The listing builds one solid part. Answer for the finished solid, in the listing's coordinates (mm). A direction names the side the tool comes from. Coordinates: 2 decimals unless noted, no trailing zeros. Write each loop counter-clockwise with the first axis right and the second up, starting at its lowest first coordinate (ties: lowest second). Pieces come first, ordered by that corner, then holes. Notation, with made-up numbers: M 42.25,-9 L 85.25,-9 A28 cw 85.25,10 Z; hole C -17,-17 d4. An arc over 180 degrees is marked long. Answer as CSV lines item,"result". Start each with the question number.
```python
from build123d import *

# Parameters (mm, degrees)
ESQUISSE1_R             = 5
BASE_EXTRUSION_DEPTH    = 9.5
ESQUISSE2_R             = 3.5
BOSS_EXTRU_1_DEPTH      = 0.5
ESQUISSE3_R             = 2.5
BOSS_EXTRU_2_DEPTH      = 14
ESQUISSE4_R             = 2
BOSS_EXTRU_3_DEPTH      = 12
CHANFREIN1_SIZE         = 0.5
CONG_1_R                = 0.5
ENL_V_MAT_EXTRU_1_DEPTH = 16
ESQUISSE9_R             = 1
ENL_V_MAT_EXTRU_2_DEPTH = 10


with BuildPart() as part:
    # Esquisse1 → Base-Extrusion (new body)
    with BuildSketch(Plane.XY):
        Circle(ESQUISSE1_R)
    extrude(amount=BASE_EXTRUSION_DEPTH)

    # Esquisse2 → Boss.-Extru.1 (add)
    with BuildSketch(Plane.XY.offset(9.5)):
        Circle(ESQUISSE2_R)
    extrude(amount=BOSS_EXTRU_1_DEPTH)

    # Esquisse3 → Boss.-Extru.2 (add)
    with BuildSketch(Plane.XY.offset(10)):
        Circle(ESQUISSE3_R)
    extrude(amount=BOSS_EXTRU_2_DEPTH)

    # Esquisse4 → Boss.-Extru.3 (add)
    with BuildSketch(Plane.XY.offset(24)):
        Circle(ESQUISSE4_R)
    extrude(amount=BOSS_EXTRU_3_DEPTH)

    # Chanfrein1
    chanfrein1_edges = [part.edges().sort_by_distance(p)[0] for p in [
        (-2, 0, 36),
    ]]
    chamfer(chanfrein1_edges, length=CHANFREIN1_SIZE)

    # Congé1
    cong_1_edges = [part.edges().sort_by_distance(p)[0] for p in [
        (-5, 0, 9.5),
    ]]
    fillet(cong_1_edges, radius=CONG_1_R)

    # Esquisse7 → Enlèv. mat.-Extru.1 (cut, symmetric)
    with BuildSketch(Plane(origin=(0, 0, 0), x_dir=(0, 0, -1), z_dir=(1, 0, 0))):
        with BuildLine():
            Line((1, 1.25), (-7, 1.25))
            ThreePointArc((-7, 1.25), (-8.25, 0), (-7, -1.25))
            Line((-7, -1.25), (1, -1.25))
            Line((1, -1.25), (1, 1.25))
        make_face()
    extrude(amount=ENL_V_MAT_EXTRU_1_DEPTH, both=True, mode=Mode.SUBTRACT)

    # Esquisse8 → Enlèvement de matière-Révolution1 (revolve, cut)
    with BuildSketch(Plane(origin=(0, 0, 0), x_dir=(0, 0, -1), z_dir=(1, 0, 0))):
        Polygon((0, 4.5), (-4, 3), (-8, 3), (-9.5, 0), (0, 0), align=None)
    revolve(axis=Axis((0, 0, 0), (0, 0, 1)), mode=Mode.SUBTRACT)

    # Esquisse9 → Enlèv. mat.-Extru.2 (cut, symmetric)
    with BuildSketch(Plane(origin=(0, 0, 0), x_dir=(1, 0, 0), z_dir=(0, 1, 0))):
        with Locations((0, -22.5)):
            Circle(ESQUISSE9_R)
    extrude(amount=ENL_V_MAT_EXTRU_2_DEPTH, both=True, mode=Mode.SUBTRACT)


solid = part.part
```
1) The part is cut by section D-D (z = 29.5). Determine the outline of the cut face in (x, y), then the cut area to 3 significant figures.
2) Which of the six approach directions +Z, -Z, +X, -X, +Y, -Y give full straight-line access (tool end or side, diameter ignored) to faces 1 (the face through (-4, -1.25, 4)), 2 (the face through (-0.064, -3.572, 2.472)), 3 (the face through (0, 0, 36)), 4 (the face through (2, -2, 10))?
3) Find the intervals of material crossed by line 1 (Z direction, x = 0, y = -1); line 2 (Y direction, x = 1.5, z = 21.5); line 3 (Z direction, x = -1.75, y = -3), in increasing order. Write a range as from..to.
4) The part is cut by section B-B (z = 15). Determine the outline of the cut face in (x, y).
5) The part is cut by section C-C (z = 22.5). Determine the outline of the cut face in (x, y), then the cut area to 3 significant figures.
6) The part is cut by section A-A (z = 7.5). Determine the outline of the cut face in (x, y).
7) Each of these flat-tipped pins is pushed along its axis until it touches: P1, Ø3, axis at y = -1.5, z = 6, coming from the -X side; P2, Ø4.5, axis at x = -1.5, y = 0.5, coming from the +Z side; P3, Ø2, axis at x = -3, y = -4, coming from the +Z side; P4, Ø6, axis at x = -0.5, z = 16, coming from the +Y side. Where does it stop, or does it pass through?
8) For a pull along Y with two mould halves and no side action, classify faces 5 (the face through (4, -1.25, 4)), 6 (the face through (1.15, -2.22, 16.9)), 7 (the face through (-0.217, 0.035, 23.476)) as +Y half, -Y half, draft (parallel to the pull), parting line (faces both ways), or undercut.
Completed:
1,outline,"C 0,0 d4"
1,area,"12.6 mm²"
2,face 1,"-Z, +X, -X"
2,face 2,"-Z"
2,face 3,"+Z, +X, -X, +Y, -Y"
2,face 4,"+Z"
3,line 1,"9..21.5, 23.5..36"
3,line 2,"-2..2"
3,line 3,"2.74..10"
4,outline,"C 0,0 d5"
5,outline,"M -1,-2.29 L -1,2.29 A2.5 ccw Z; M 1,-2.29 A2.5 ccw 1,2.29 Z"
5,area,"9.91 mm²"
6,outline,"M -4.87,-1.15 A5 ccw 4.87,-1.15 L 2.77,-1.15 A3 cw -2.77,-1.15 Z; M -4.87,1.15 L -2.77,1.15 A3 cw 2.77,1.15 L 4.87,1.15 A5 ccw Z"
7,P1,"x = -4.86"
7,P2,"z = 36"
7,P3,"z = 9.5"
7,P4,"y = 2.5"
8,face 5,"undercut"
8,face 6,"parting line"
8,face 7,"draft"
